Input: part model. Units: mm. Frame: model coordinates. Coordinates: 2 decimals unless noted, no trailing zeros. Loops run counter-clockwise (first coordinate to the right, second up) from the corner with the lowest first, then second, coordinate; pieces in that order, holes last. Notation, with made-up numbers: (28, 86.25) - (83, 86.25) arc R22 cw to (83, 92.25) - close; hole circle Ø4 at (17.25, -22.75). An arc over 180 degrees is marked (long way). Use one line per item in the form item = value.
from build123d import *

# Parameters (mm, degrees)
BOSS_EXTRUDE1_DEPTH             = 6.35
F_1_4_CLEARANCE_HOLE1_D         = 6.7564
CUT_EXTRUDE1_DEPTH              = 929.886717725
FILLET1_R                       = 3.175
SKETCH5_W                       = 44.45
SKETCH5_H                       = 76.2
BOSS_EXTRUDE2_DEPTH             = 6.35
FILLET2_R                       = 2.54
F_1_4_0_25_DIAMETER_SLOT1_DEPTH = 6.35
F_5_16_0_3125_DIAMETER_HOLE1_D  = 7.9375


# Read off the part's stored shape, not the designer's step: 1/4 (0.25) Diameter Slot1
with BuildPart() as part:
    # Sketch1 → Boss-Extrude1 (new body)
    with BuildSketch(Plane(origin=(0, 0, 0), x_dir=(0, 0, -1), z_dir=(1, 0, 0))):
        with BuildLine():
            Line((0, 19.05), (50.8, 19.05))
            ThreePointArc((50.8, 19.05), (269.697199621, -83.023440532), (332.208815423, -316.319966768))
            Line((332.208815423, -316.319966768), (281.874321133, -601.781069134))
            ThreePointArc((281.874321133, -601.781069134), (280.337795232, -613.452142071), (279.824317306, -625.212720108))
            Line((279.824317306, -625.212720108), (279.824317306, -865.750720108))
            Line((279.824317306, -865.750720108), (44.45, -865.750720108))
            Line((44.45, -865.750720108), (44.45, -674.7002))
            Line((44.45, -674.7002), (0, -674.7002))
            Line((0, -674.7002), (0, -605.1296))
            Line((0, -605.1296), (38.1, -605.1296))
            Line((38.1, -605.1296), (38.1, -534.7716))
            Line((38.1, -534.7716), (0, -534.7716))
            Line((0, -534.7716), (0, 19.05))
        make_face()
    extrude(amount=BOSS_EXTRUDE1_DEPTH)

    # 1/4 Clearance Hole1 (through all)
    with Locations(Plane(origin=(6.35, 0, 0), x_dir=(0, 0, -1), z_dir=(1, 0, 0))):
        with Locations((25.4, 9.525), (262.400626301, -89.145992514), (321.450189166, -322.482879416), (270.849040732, -612.621983621), (270.299317306, -840.350720108), (38.1, -639.9149), (38.1, -422.275), (76.2, -637.430120108), (228.6, -637.430120108), (76.2, -856.225720108), (228.6, -856.225720108), (228.6, -618.380120108), (76.2, -618.380120108), (57.15, -789.550720108)):
            Hole(F_1_4_CLEARANCE_HOLE1_D / 2)

    # Sketch4 → Cut-Extrude1 (cut, through all)
    with BuildSketch(Plane(origin=(6.35, 0, 0), x_dir=(0, 0, -1), z_dir=(1, 0, 0))):
        with BuildLine():
            Line((50.8, -0.79375), (12.7, -0.79375))
            ThreePointArc((12.7, -0.79375), (11.1125, 0.79375), (12.7, 2.38125))
            Line((12.7, 2.38125), (50.8, 2.38125))
            ThreePointArc((50.8, 2.38125), (52.3875, 0.79375), (50.8, -0.79375))
        make_face()
        with BuildLine():
            Line((313.863635816, -324.369144862), (300.080311714, -402.538260258))
            ThreePointArc((300.080311714, -402.538260258), (298.241262924, -403.825976083), (296.953547098, -401.986927293))
            Line((296.953547098, -401.986927293), (310.7368712, -323.817811898))
            ThreePointArc((310.7368712, -323.817811898), (312.57591999, -322.530096072), (313.863635816, -324.369144862))
        make_face()
        with BuildLine():
            Line((267.388472275, -587.942894917), (281.171796377, -509.773779521))
            ThreePointArc((281.171796377, -509.773779521), (279.884080551, -507.934730732), (278.045031761, -509.222446557))
            Line((278.045031761, -509.222446557), (264.261707659, -587.391561953))
            ThreePointArc((264.261707659, -587.391561953), (265.549423485, -589.230610743), (267.388472275, -587.942894917))
        make_face()
        with BuildLine():
            Line((259.980567306, -803.838220108), (259.980567306, -699.063220108))
            ThreePointArc((259.980567306, -699.063220108), (261.568067306, -697.475720108), (263.155567306, -699.063220108))
            Line((263.155567306, -699.063220108), (263.155567306, -803.838220108))
            ThreePointArc((263.155567306, -803.838220108), (261.568067306, -805.425720108), (259.980567306, -803.838220108))
        make_face()
    extrude(amount=-CUT_EXTRUDE1_DEPTH, mode=Mode.SUBTRACT)

    # Fillet1
    fillet1_edges = [part.edges().sort_by_distance(p)[0] for p in [
        (3.175, -605.1296, -38.1),
        (3.175, -534.7716, -38.1),
        (3.175, -534.7716, 0),
        (3.175, 19.05, 0),
        (3.175, -865.750720108, -279.824317306),
        (3.175, -865.750720108, -44.45),
        (3.175, -674.7002, -44.45),
        (3.175, -674.7002, 0),
        (3.175, -605.1296, 0),
    ]]
    fillet(fillet1_edges, radius=FILLET1_R)

    # Sketch5 → Boss-Extrude2 (add)
    with BuildSketch(Plane(origin=(6.35, 0, 0), x_dir=(0, 0, -1), z_dir=(1, 0, 0))):
        with Locations((22.225, -789.0002)):
            Rectangle(SKETCH5_W, SKETCH5_H)
    extrude(amount=-BOSS_EXTRUDE2_DEPTH)

    # Fillet2
    fillet2_edges = [part.edges().sort_by_distance(p)[0] for p in [
        (3.175, -750.9002, -44.45),
        (3.175, -827.1002, -44.45),
        (3.175, -827.1002, 0),
        (3.175, -750.9002, 0),
    ]]
    fillet(fillet2_edges, radius=FILLET2_R)

    # 1/4 (0.25) Diameter Slot1 outline → 1/4 (0.25) Diameter Slot1 (cut)
    with BuildSketch(Plane.YZ):
        with BuildLine():
            Line((-786.375720108, -38.1), (-786.375720108, -25.4))
            ThreePointArc((-786.375720108, -25.4), (-789.550720108, -22.225), (-792.725720108, -25.4))
            Line((-792.725720108, -25.4), (-792.725720108, -38.1))
            ThreePointArc((-792.725720108, -38.1), (-789.550720108, -41.275), (-786.375720108, -38.1))
        make_face()
    extrude(amount=F_1_4_0_25_DIAMETER_SLOT1_DEPTH, mode=Mode.SUBTRACT)

    # 5/16 (0.3125) Diameter Hole1 (through all)
    with Locations(Plane(origin=(6.35, 0, 0), x_dir=(0, 0, -1), z_dir=(1, 0, 0))):
        with Locations((15.875, -522.0716), (15.875, -617.8296)):
            Hole(F_5_16_0_3125_DIAMETER_HOLE1_D / 2)


solid = part.part
Q1. First-contact query: P1, Ø3, axis at x = 4.5, z = -34.5, coming from the -Y side; P2, Ø1, axis at x = 5.5, y = -584.5, coming from the +Z side; P3, Ø5.5, axis at y = -789.55, z = -57.15, coming from the +X side; P4, Ø3, axis at x = 4, y = -726, coming from the +Z side. Flat tips, straight axial feed; report the tip coordinate or a pass-through.
Check values:
P1 = -827.1
P2 = -38.1
P3 = through
P4 = -44.45
Q2. Cut plane B-B, the plane x = 2.5. Give the number of separate pieces and of enclosed holes in the cut face, then the cut area to 3 significant figures.
Check values:
separate_pieces = 1
enclosed_holes = 21
area = 247,000 mm²
Q3. Cut plane A-A, the plane z = -139.5. Return loops of the section in (x, y).
Check values:
outline = (0, -865.75) - (6.35, -865.75) - (6.35, 4.93) - (0, 4.93) - close
Q4. Cut plane C-C, the plane y = -209. Return loops of the section in (x, z).
Check values:
outline = (0, -330.66) - (6.35, -330.66) - (6.35, 0) - (0, 0) - close
Q5. Ray query, line 1 along Y through (x, z) = (3.25, -25.4); line 2 along Y through (x, z) = (2, -57.15); line 3 along Z through (x, y) = (3.75, -720.5). Return the intervals inside material, ascending. Write a range as [from, to].
Check values:
line_1 = [-827.1, -792.73], [-786.38, -750.9], [-674.7, -605.13], [-534.77, -0.79], [2.38, 6.15], [12.9, 19.05]
line_2 = [-865.75, -792.93], [-786.17, 18.98]
line_3 = [-279.82, -263.16], [-259.98, -44.45]
